For this review, take the finished solid that the model builds, in its own axes (mm). A direction names the side the tool comes from. Coordinates: 2 decimals unless noted, no trailing zeros. Write each loop counter-clockwise with the first axis right and the second up, starting at its lowest first coordinate (ties: lowest second). Pieces come first, ordered by that corner, then holes.
```python
from build123d import *

# Parameters (mm, degrees)
SKETCH1_R                       = 2.25
BOSS_EXTRUDE1_DEPTH             = 3.175
F_8_32_TAPPED_HOLE1_D           = 3.4544
F_8_32_TAPPED_HOLE1_DEPTH       = 10.71
F_8_32_TAPPED_HOLE1_TIP         = 1.037806461
F_3_16_0_1875_DOWEL_HOLE1_D     = 4.7625
F_3_16_0_1875_DOWEL_HOLE1_DEPTH = 12.83
F_3_16_0_1875_DOWEL_HOLE1_TIP   = 1.430799349
FILLET1_R                       = 25


with BuildPart() as part:
    # Sketch1 → Boss-Extrude1 (new, symmetric)
    with BuildSketch(Plane(origin=(0, 0, 0), x_dir=(1, 0, 0), z_dir=(0, 1, 0))):
        Polygon((80.256619665, -122.683026536), (8.485281374, -26.870057685), (1.414213562, -19.798989873), (19.798989873, -1.414213562), (26.870057685, -8.485281374), (122.683026536, -80.256619665), align=None)
        with Locations(Location((8.485281374, -19.798989873, 0), (0, 0, 270))):
            Circle(SKETCH1_R, mode=Mode.SUBTRACT)
        with Locations(Location((19.798989873, -8.485281374, 0), (0, 0, 270))):
            Circle(SKETCH1_R, mode=Mode.SUBTRACT)
    extrude(amount=BOSS_EXTRUDE1_DEPTH, both=True)

    # #8-32 Tapped Hole1
    with Locations(Plane(origin=(101.4698231, 0, 101.4698231), x_dir=(0.7071067811865462, 0, -0.7071067811865489), z_dir=(0.7071067811865489, 0, 0.7071067811865462))):
        with Locations((20, 0), (-20, 0)):
            Hole(F_8_32_TAPPED_HOLE1_D / 2, depth=F_8_32_TAPPED_HOLE1_DEPTH)
            with Locations((0, 0, -(F_8_32_TAPPED_HOLE1_DEPTH + F_8_32_TAPPED_HOLE1_TIP / 2))):  # 118° drill point
                Cone(0, F_8_32_TAPPED_HOLE1_D / 2, F_8_32_TAPPED_HOLE1_TIP, mode=Mode.SUBTRACT)

    # 3/16 (0.1875) Dowel Hole1
    with Locations(Plane(origin=(101.4698231, 0, 101.4698231), x_dir=(0.7071067811865462, 0, -0.7071067811865489), z_dir=(0.7071067811865489, 0, 0.7071067811865462))):
        with Locations((-10, 0), (10, 0)):
            Hole(F_3_16_0_1875_DOWEL_HOLE1_D / 2, depth=F_3_16_0_1875_DOWEL_HOLE1_DEPTH)
            with Locations((0, 0, -(F_3_16_0_1875_DOWEL_HOLE1_DEPTH + F_3_16_0_1875_DOWEL_HOLE1_TIP / 2))):  # 118° drill point
                Cone(0, F_3_16_0_1875_DOWEL_HOLE1_D / 2, F_3_16_0_1875_DOWEL_HOLE1_TIP, mode=Mode.SUBTRACT)

    # Fillet1
    fillet1_edges = [part.edges().sort_by_distance(p)[0] for p in [
        (8.485281374, 0, 26.870057685),
        (26.870057685, 0, 8.485281374),
    ]]
    fillet(fillet1_edges, radius=FILLET1_R)


solid = part.part
```
1) For L1, parallel to Z at x = 105.5, y = -1.5; L2, parallel to X at y = 1, z = 112; L3, parallel to Z at x = 81.5, y = -0.75, list the stretches that pass through material, from the lowest coordinate up.
2) Tool access review of faces 1 (the face through (98.9, -0.16, 84.22)), 2 (the face through (62, -3.175, 62)): name each direction out of +Z, -Z, +X, -X, +Y, -Y from which nothing blocks a thin tool from reaching the whole face with its end or side.
3) The part is to be moulded in two halves that separate along Z. For faces 3 (the face through (8.454, -0.044, 26.931)), 4 (the face through (6.49, -0.04, 20.84)), 5 (the face through (102.386, -0.912, 91.355)), 6 (the face through (26.931, 0.044, 8.454)), say which applies: pulls with the +Z half, pulls with the -Z half, needs draft (parallel to the pull), parting line crosses it, or undercut.
4) Consider section A-A (z = 66.5). Give the boundary of the cut face in (x, y) (3 decimals), then the cut area to 3 significant figures.
5) Consider section B-B (x = 73). Give the boundary of the cut face in (y, z) (3 decimals).
6) Clearance check with flat-ended pins moving along their axes: P1, Ø1.5, axis at x = 107.5, y = -0.5, coming from the +Z side; P2, Ø1, axis at x = 57, y = -1, coming from the -Z side; P3, Ø5, axis at x = 19.8, z = 8.49, coming from the +Y side (3 decimals). State where each tip first meets the part, or that it passes through.
Results:
1. L1: z = 67.39 to 88.74, 93.97 to 97.44
1. L2: x = 72.25 to 81.72, 85.71 to 90.94
1. L3: z = 49.41 to 107.58, 111.98 to 121.44
2. face 1: none
2. face 2: +Z, -Z, +X, -X, -Y
3. face 3: pulls with the +Z half
3. face 4: undercut
3. face 5: undercut
3. face 6: pulls with the -Z half
4. outline: (38.171, -3.175) - (104.318, -3.175) - (104.318, 3.175) - (38.171, 3.175) - close
4. area: 420 mm2
5. outline: (-3.175, 43.04) - (3.175, 43.04) - (3.175, 112.996) - (-3.175, 112.996) - close
6. P1: stops at z = 96.19
6. P2: stops at z = 30.68
6. P3: stops at y = 3.175
